Could you check a few things on this model? Use its own coordinates, in mm. A direction names the side the tool comes from. Coordinates: 2 decimals unless noted, no trailing zeros. Loops run counter-clockwise (first coordinate to the right, second up) from the corner with the lowest first, then second, coordinate; pieces in that order, holes last. Notation, with made-up numbers: (39.25, 84) - (59.25, 84) arc R19 ccw to (59.25, 113) - close; hole circle Ø7 at (-13.5, 45.25). An arc over 180 degrees is marked (long way). One line per question, with ' | ' between items. Start each with the question number.
1. I want a section at B-B, the plane z = 26. Write out the boundary of the cut face in (x, y) (3 decimals), then the cut area to 3 significant figures.
2. I want a section at A-A, the plane y = 17. Write out the boundary of the cut face in (x, z) (3 decimals).
3. I want a section at D-D, the plane z = 31.75. Write out the boundary of the cut face in (x, y) (3 decimals), then the cut area to 3 significant figures.
4. Which directions (+Z, -Z, +X, -X, +Y, -Y) give clear straight access to the entire face, cutting with the end or side of a thin tool? Please do faces 1 (the flat face through (1.625, -2, 30)), 2 (the flat face through (1, -65.371, 30)).
5. I want a section at C-C, the plane y = 37. Write out the boundary of the cut face in (x, z) (3 decimals).
6. We'd pull the mould along Z, two halves only. Please class faces 3 (the flat face through (5, -1, 30)), 4 (the flat face through (3.375, -2, 30)), 5 (the flat face through (2, -1, 19.146)), 6 (the cylindrical face through (2.465, 53.663, 35.185)): pulls with the +Z half, pulls with the -Z half, needs draft (parallel to the pull), parting line crosses it, or undercut.
7. Please list where these lines run through material, in increasing order: L1, parallel to X at y = -38.5, z = 21.75 (3 decimals); L2, parallel to Z at x = 2.95, y = -53.5; L3, parallel to Z at x = 2.95, y = 38. Write a range as [from, to].
from build123d import *

# Parameters (mm, degrees)
F0_W        = 130
F0_H        = 22
F1_DEPTH    = 5
F2_T1_DEPTH = 149.568322948
F3_T        = -1.625


# Not quite as in the source:
# - a fillet or chamfer that OpenCascade refuses, or shapes differently, is made with other operations: its cross-section is extruded or revolved along the edge and cut away or added


with BuildPart() as f1:
    # F0 (on Right) → F1 (new body)
    with BuildSketch(Plane.YZ):
        with Locations((-0.3712646805, 30.1455706358)):
            Rectangle(F0_W, F0_H)
    extrude(amount=F1_DEPTH)

    # F2: fillet of radius 30 on 1 edges, made by hand

    # F2_s2 → F2_t1 (cut)
    with BuildSketch(Plane.YZ.offset(-72.284161474)):
        with BuildLine():
            ThreePointArc((35.7150707299, 41.1455706358), (53.8809728545, 35.0202434084), (64.6287353195, 19.1455706358))
            Line((64.6287353195, 19.1455706358), (64.6287353195, 41.1455706358))
            Line((64.6287353195, 41.1455706358), (35.7150707299, 41.1455706358))
        make_face()
    extrude(amount=F2_T1_DEPTH, mode=Mode.SUBTRACT)

    # F3
    f3_openings = [f1.faces().sort_by_distance(p)[0] for p in [
        (2.5, -65.371265, 30.145571),
    ]]
    offset(amount=F3_T, openings=f3_openings)


solid = f1.part
Results are:
1) outline: (0, -65.371) - (1.625, -65.371) - (1.625, 59.891) - (3.375, 59.891) - (3.375, -65.371) - (5, -65.371) - (5, 61.779) - (0, 61.779) - close | area: 417 mm2
2) outline: (0, 19.146) - (5, 19.146) - (5, 41.146) - (0, 41.146) - close; hole (1.625, 20.771) - (3.375, 20.771) - (3.375, 39.521) - (1.625, 39.521) - close
3) outline: (0, -65.371) - (1.625, -65.371) - (1.625, 55.224) - (3.375, 55.224) - (3.375, -65.371) - (5, -65.371) - (5, 57.52) - (0, 57.52) - close | area: 403 mm2
4) face 1: -Y | face 2: +Z, -Z, +X, -X, -Y
5) outline: (0, 19.146) - (5, 19.146) - (5, 41.118) - (0, 41.118) - close; hole (1.625, 20.771) - (3.375, 20.771) - (3.375, 39.491) - (1.625, 39.491) - close
6) face 3: needs draft | face 4: undercut | face 5: pulls with the -Z half | face 6: pulls with the +Z half
7) L1: x = [0, 1.625], [3.375, 5] | L2: z = [19.15, 20.77], [39.52, 41.15] | L3: z = [19.15, 20.77], [39.43, 41.06]
